from build123d import *

# Parameters (mm, degrees)
SKETCH_1_R          = 3.5
EXTRUDE_1_DEPTH     = 54.5
SKETCH_2_R          = 1
CUT_EXTRUDE_2_DEPTH = 27.25
SKETCH_3_R          = 7.070877384
CUT_EXTRUDE_3_DEPTH = 3
SKETCH_4_R          = 6.045504862
CUT_EXTRUDE_4_DEPTH = 4


with BuildPart() as part:
    # Эскиз1 → Вытянуть1 (new body)
    with BuildSketch(Plane(origin=(0, 0, 0), x_dir=(1, 0, 0), z_dir=(0, 1, 0))):
        with Locations(Location((0, 0, 0), (0, 0, 270))):
            Circle(SKETCH_1_R)
    extrude(amount=EXTRUDE_1_DEPTH)

    # Эскиз2 → Вытянуть2 (cut, symmetric)
    with BuildSketch(Plane.XY):
        with Locations(Location((0, 48.5, 0), (0, 0, 89.99999997))):
            Circle(SKETCH_2_R)
        with Locations(Location((0, 7, 0), (0, 0, 89.99999997))):
            Circle(SKETCH_2_R)
    extrude(amount=CUT_EXTRUDE_2_DEPTH, both=True, mode=Mode.SUBTRACT)

    # Эскиз3 → Вытянуть3 (cut)
    with BuildSketch(Plane(origin=(0, 54.5, 0), x_dir=(1, 0, 0), z_dir=(0, 1, 0))):
        Circle(SKETCH_3_R)
    extrude(amount=-CUT_EXTRUDE_3_DEPTH, mode=Mode.SUBTRACT)

    # Эскиз4 → Вытянуть4 (cut)
    with BuildSketch(Plane.XZ):
        Circle(SKETCH_4_R)
    extrude(amount=-CUT_EXTRUDE_4_DEPTH, mode=Mode.SUBTRACT)


solid = part.part
Design review of the part built by this model. Coordinates are the model's own, in mm. Give positions to 0.01 mm unless a question says otherwise; leave off trailing zeros. Order: outer loops, then holes, each group sorted by start corner. A loop starts at its lowest first (then second) coordinate and runs counter-clockwise, first axis right, second up. Notation, with made-up numbers: (29, 9) - (54, 9) arc R20 ccw to (54, 48) - close; hole circle Ø7 at (-28, 86.25). An arc over 180 degrees is marked (long way). Write item = value, one per line. Start each with the question number.
Q1. We need section A-A on x = 0. State the section outline as (y, z) points, plus the area to 4 significant figures.
Q2. We need section B-B on z = -1.25. State the section outline as (x, y) points, plus the area to 3 significant figures.
Q3. Clearance check with flat-ended pins moving along their axes: pin 1 Ø1.5 at (x, y) = (1, 40.5) entering from -Z; pin 2 Ø1 at (y, z) = (13.5, 2.5) entering from +X; pin 3 Ø1.5 at (y, z) = (18, 2) entering from -X. State where each tip first meets the part, or that it passes through.
Q4. We need section D-D on y = 7. State the section outline as (x, z) points.
Q5. We need section C-C on y = 45.5. State the section outline as (x, z) points, plus the area to 3 significant figures.
Q6. Mouldability with a two-part tool opening along X and no side actions: class faces 1 (the face through (0, 6, 0)), 2 (the face through (0, 51.5, 0)), 3 (the face through (-1.341, 27.418, 3.233)) as released by +X, released by -X, zero draft, split by the parting line, or undercut.
Q7. To check wall thickness, follow L1, parallel to Y at x = 0.5, z = 3; L2, parallel to Z at x = 0.25, y = 16.5; L3, parallel to X at y = 29.5, z = -2.5. State the ranges of each line that lie inside material, in increasing order. Write a range as from..to.
Working result:
q1.outline = (4, -3.5) - (6, -3.5) - (6, 3.5) - (4, 3.5) - close; (8, -3.5) - (47.5, -3.5) - (47.5, 3.5) - (8, 3.5) - close; (49.5, -3.5) - (51.5, -3.5) - (51.5, 3.5) - (49.5, 3.5) - close
q1.area = 304.5 mm²
q2.outline = (-3.27, 4) - (3.27, 4) - (3.27, 51.5) - (-3.27, 51.5) - close; hole circle Ø2 at (0, 7); hole circle Ø2 at (0, 48.5)
q2.area = 304 mm²
q3.pin_1 = -3.49
q3.pin_2 = 2.87
q3.pin_3 = -3.27
q4.outline = (-1, -3.35) - (-1, 3.35) arc R3.5 ccw to start; (1, -3.35) arc R3.5 ccw to (1, 3.35) - close
q5.outline = circle Ø7 at (0, 0)
q5.area = 38.5 mm²
q6.face_1 = undercut
q6.face_2 = zero draft
q6.face_3 = split by the parting line
q7.L1 = 4..6.13, 7.87..47.63, 49.37..51.5
q7.L2 = -3.49..3.49
q7.L3 = -2.45..2.45
